from build123d import *

# Parameters (mm, degrees)
PRISM_DEPTH       = 2.4
PRISM001_DEPTH    = 2.4
CYLINDER012_R     = 1.25
CYLINDER012_DEPTH = 50
CYLINDER011_R     = 1.25
CYLINDER011_DEPTH = 50
CYLINDER007_R     = 6.75
CYLINDER007_DEPTH = 50
CYLINDER008_R     = 6.75
CYLINDER008_DEPTH = 50
BOX002_W          = 18
BOX002_H          = 18
BOX002_DEPTH      = 15
BOX003_W          = 18
BOX003_H          = 18
BOX003_DEPTH      = 15
CYLINDER004_R     = 11.2
CYLINDER004_DEPTH = 23
CYLINDER002_R     = 0.9
CYLINDER002_DEPTH = 19.75
ARRAY001_COUNT    = 10
CYLINDER006_R     = 10.5
CYLINDER006_DEPTH = 32
CYLINDER005_R     = 20
CYLINDER005_DEPTH = 15
FILLET003_R       = 1
CYLINDER029_R     = 1.25
CYLINDER029_DEPTH = 50
BOX009_W          = 16
BOX009_H          = 1
BOX009_DEPTH      = 15
CYLINDER030_R     = 1.25
CYLINDER030_DEPTH = 50
BOX010_W          = 16
BOX010_H          = 1
BOX010_DEPTH      = 15
FILLET010_R       = 0.9


with BuildPart() as prism:
    # Prism → Prism (new body)
    with BuildSketch(Plane(origin=(0, 28, 22.5), x_dir=(1, 0, 0), z_dir=(0, -1, 0))):
        Polygon((3.15, 0), (1.575, 2.72798), (-1.575, 2.72798), (-3.15, 0), (-1.575, -2.72798), (1.575, -2.72798), align=None)
    extrude(amount=PRISM_DEPTH)


with BuildPart() as prism001:
    # Prism001 → Prism001 (new body)
    with BuildSketch(Plane(origin=(0, -25.5, 22.5), x_dir=(1, 0, 0), z_dir=(0, -1, 0))):
        Polygon((3.15, 0), (1.575, 2.72798), (-1.575, 2.72798), (-3.15, 0), (-1.575, -2.72798), (1.575, -2.72798), align=None)
    extrude(amount=PRISM001_DEPTH)


with BuildPart() as cylinder011:
    # Cylinder012 → Cylinder012 (new body)
    with BuildSketch(Plane(origin=(0, 69, 22.5), x_dir=(1, 0, 0), z_dir=(0, -1, 0))):
        Circle(CYLINDER012_R)
    extrude(amount=CYLINDER012_DEPTH)


with BuildPart() as cylinder010:
    # Cylinder011 → Cylinder011 (new body)
    with BuildSketch(Plane(origin=(0, -16, 22.5), x_dir=(1, 0, 0), z_dir=(0, -1, 0))):
        Circle(CYLINDER011_R)
    extrude(amount=CYLINDER011_DEPTH)


with BuildPart() as cylinder007:
    # Cylinder007 → Cylinder007 (new body)
    with BuildSketch(Plane(origin=(-24, 19, 22.5), x_dir=(0, 0, -1), z_dir=(1, 0, 0))):
        Circle(CYLINDER007_R)
    extrude(amount=CYLINDER007_DEPTH)


with BuildPart() as cylinder008:
    # Cylinder008 → Cylinder008 (new body)
    with BuildSketch(Plane(origin=(-24, -19, 22.5), x_dir=(0, 0, -1), z_dir=(1, 0, 0))):
        Circle(CYLINDER008_R)
    extrude(amount=CYLINDER008_DEPTH)


with BuildPart() as cube002:
    # Box002 → Box002 (new body)
    with BuildSketch(Plane(origin=(-9, -29, 15), x_dir=(1, 0, 0), z_dir=(0, 0, 1))):
        with Locations((9, 9)):
            Rectangle(BOX002_W, BOX002_H)
    extrude(amount=BOX002_DEPTH)


with BuildPart() as cube003:
    # Box003 → Box003 (new body)
    with BuildSketch(Plane(origin=(-9, 11, 15), x_dir=(1, 0, 0), z_dir=(0, 0, 1))):
        with Locations((9, 9)):
            Rectangle(BOX003_W, BOX003_H)
    extrude(amount=BOX003_DEPTH)


with BuildPart() as cylinder004:
    # Cylinder004 → Cylinder004 (new body)
    with BuildSketch(Plane.XY):
        Circle(CYLINDER004_R)
    extrude(amount=CYLINDER004_DEPTH)


with BuildPart() as obj1:
    # Cylinder002 → Cylinder002 (new body)
    with BuildSketch(Plane(origin=(0, 0, 15), x_dir=(0, 0, -1), z_dir=(1, 0, 0))):
        Circle(CYLINDER002_R)
    extrude(amount=CYLINDER002_DEPTH)

    # Array001: obj1 ×10 about axis
    array001_axis = Axis((0, 0, 0), (0, 0, 1))


with BuildPart() as obj1_1:
    add(obj1.part)
    for i in range(1, ARRAY001_COUNT):
        add(obj1.part.rotate(array001_axis, i * 360 / ARRAY001_COUNT))

    # Cut002: cut Cylinder004
    add(cylinder004.part, mode=Mode.SUBTRACT)


with BuildPart() as cylinder006:
    # Cylinder006 → Cylinder006 (new body)
    with BuildSketch(Plane.XY):
        Circle(CYLINDER006_R)
    extrude(amount=CYLINDER006_DEPTH)


with BuildPart() as obj2:
    # Cylinder005 → Cylinder005 (new body)
    with BuildSketch(Plane.XY.offset(15)):
        Circle(CYLINDER005_R)
    extrude(amount=CYLINDER005_DEPTH)

    # Cut004: cut Cylinder006
    add(cylinder006.part, mode=Mode.SUBTRACT)

    # Fusion001: union obj1
    add(obj1_1.part)

    # Fusion002: union Cube002, Cube003
    add(cube002.part)
    add(cube003.part)

    # Cut005: cut Cylinder008
    add(cylinder008.part, mode=Mode.SUBTRACT)

    # Cut006: cut Cylinder007
    add(cylinder007.part, mode=Mode.SUBTRACT)

    # Fillet003
    fillet003_edges = [obj2.edges().sort_by_distance(p)[0] for p in [
        (-9, -17.860571, 29.576567),
        (-9, -17.860571, 15.423433),
        (-9, -29, 22.5),
        (-9, 17.860571, 15.423433),
        (-9, 17.860571, 29.576567),
        (9, -29, 22.5),
        (9, -17.860571, 29.576567),
        (9, -17.860571, 15.423433),
        (9, 17.860571, 29.576567),
        (9, 17.860571, 15.423433),
        (9, 29, 22.5),
        (-9, 29, 22.5),
    ]]
    fillet(fillet003_edges, radius=FILLET003_R)

    # Cut008: cut Cylinder010
    add(cylinder010.part, mode=Mode.SUBTRACT)

    # Cut009: cut Cylinder011
    add(cylinder011.part, mode=Mode.SUBTRACT)

    # Cut025: cut Prism001
    add(prism001.part, mode=Mode.SUBTRACT)

    # Cut026: cut Prism
    add(prism.part, mode=Mode.SUBTRACT)


with BuildPart() as cylinder020:
    # Cylinder029 → Cylinder029 (new body)
    with BuildSketch(Plane(origin=(0, 69, 22.5), x_dir=(1, 0, 0), z_dir=(0, -1, 0))):
        Circle(CYLINDER029_R)
    extrude(amount=CYLINDER029_DEPTH)


with BuildPart() as cut027:
    # Box009 → Box009 (new body)
    with BuildSketch(Plane(origin=(-8, 29, 15), x_dir=(1, 0, 0), z_dir=(0, 0, 1))):
        with Locations((8, 0.5)):
            Rectangle(BOX009_W, BOX009_H)
    extrude(amount=BOX009_DEPTH)

    # Cut027: cut Cylinder020
    add(cylinder020.part, mode=Mode.SUBTRACT)


with BuildPart() as cylinder021:
    # Cylinder030 → Cylinder030 (new body)
    with BuildSketch(Plane(origin=(0, 69, 22.5), x_dir=(1, 0, 0), z_dir=(0, -1, 0))):
        Circle(CYLINDER030_R)
    extrude(amount=CYLINDER030_DEPTH)


with BuildPart() as obj3:
    # Box010 → Box010 (new body)
    with BuildSketch(Plane(origin=(-8, 29, 15), x_dir=(1, 0, 0), z_dir=(0, 0, 1))):
        with Locations((8, 0.5)):
            Rectangle(BOX010_W, BOX010_H)
    extrude(amount=BOX010_DEPTH)

    # Cut028: cut Cylinder021
    add(cylinder021.part, mode=Mode.SUBTRACT)


with BuildPart() as obj3_1:
    # Cut028 placement: moved
    add(obj3.part.moved(Location((0, -59, 0))))

    # Fusion008: union obj2, Cut027
    add(obj2.part)
    add(cut027.part)

    # Fillet010
    fillet010_edges = [obj3_1.edges().sort_by_distance(p)[0] for p in [
        (-8, -30, 22.5),
        (8, -30, 22.5),
        (-8, 30, 22.5),
        (8, 30, 22.5),
    ]]
    fillet(fillet010_edges, radius=FILLET010_R)


solid = obj3_1.part
Check sheet for the modelled part. Datum: model origin and axes. Units: mm. A direction names the side the tool comes from. Round coordinates to 2 decimals unless told otherwise and drop trailing zeros. Loops run counter-clockwise (first coordinate to the right, second up) from the corner with the lowest first, then second, coordinate; pieces in that order, holes last. Notation, with made-up numbers: M -14.75,73.5 L 19.25,73.5 A26 ccw 19.25,97.5 Z; hole C 70.5,7 d7. An arc over 180 degrees is marked long. One line per item, written item: value.
(1) Thickness scan on line 1 (X direction, y = 29.05, z = 22.5); line 2 (Z direction, x = -2.5, y = -19); line 3 (Y direction, x = 0, z = 25). Record the ranges inside material, lowest first.
Computed values:
line 1: x = -8 to -1.25, 1.25 to 8
line 2: z = 15 to 15.75, 29.25 to 30
line 3: y = -30 to -27.9, -25.5 to -25.27, -12.73 to -10.5, 10.5 to 12.73, 25.27 to 25.6, 28 to 30
(2) Sectioned sample at C-C, the plane y = 26.5. Record the cut outline in (x, z) (3 decimals), then the cut area to 3 significant figures.
Computed values:
outline: M -9,15 L 9,15 L 9,30 L -9,30 Z; hole M -3.15,22.5 L -1.575,19.772 L 1.575,19.772 L 3.15,22.5 L 1.575,25.228 L -1.575,25.228 Z
area: 244 mm^2
(3) Depth check by flat-ended pin: pin 1 Ø1.9 at (x, y) = (0, 27.5) entering from -Z; pin 2 Ø4 at (x, z) = (13, 28.5) entering from -Y; pin 3 Ø1.5 at (x, z) = (0, 22.5) entering from -Y; pin 4 Ø8 at (y, z) = (-3, 20.5) entering from +X. Enter the tip coordinate at first touch or a pass-through.
Computed values:
pin 1: stops at z = 15
pin 2: stops at y = -16.68
pin 3: stops at y = -12.29
pin 4: stops at x = 20
(4) Sectioned sample at B-B, the plane y = 0. Record the cut outline in (x, z).
Computed values:
outline: M -20,15 L -19.75,15 L -19.75,14.1 L -11.2,14.1 L -11.2,15 L -10.5,15 L -10.5,30 L -20,30 Z; M 10.5,15 L 11.2,15 L 11.2,14.1 L 19.75,14.1 L 19.75,15 L 20,15 L 20,30 L 10.5,30 Z
(5) Release check for a two-part mould opening along Y. For faces 5 (the face through (9, 26, 22)), 6 (the face through (-2, 30, 22)), 7 (the face through (-4.8, -14.6, 14.1)) record: +Y half, -Y half, draft (parallel to the pull), parting line (faces both ways), or undercut.
Computed values:
face 5: draft
face 6: +Y half
face 7: undercut
(6) Sectioned sample at A-A, the plane x = 0. Record the cut outline in (y, z), then the cut area to 3 significant figures.
Computed values:
outline: M -30,15 L -10.5,15 L -10.5,30 L -30,30 L -30,23.75 L -27.9,23.75 L -27.9,25.23 L -25.5,25.23 L -25.5,24.32 A6.75 cw long -25.5,20.68 L -25.5,19.77 L -27.9,19.77 L -27.9,21.25 L -30,21.25 Z; M 10.5,15 L 30,15 L 30,21.25 L 28,21.25 L 28,19.77 L 25.6,19.77 L 25.6,21.08 A6.75 cw long 25.6,23.92 L 25.6,25.23 L 28,25.23 L 28,23.75 L 30,23.75 L 30,30 L 10.5,30 Z
area: 263 mm^2
(7) Sectioned sample at D-D, the plane y = -22. Record the cut outline in (x, z).
Computed values:
outline: M -9,15 L 9,15 L 9,16.45 L -9,16.45 Z; M -9,28.55 L 9,28.55 L 9,30 L -9,30 Z
(8) Access from +Z, -Z, +X, -X, +Y, -Y to the whole of each face (thin tool, end or side, straight path). Record for faces 1 (the face through (9, -26, 22)), 2 (the face through (-2.4, -26.7, 21.2)), 3 (the face through (-4.7, 14.6, 14.1)), 4 (the face through (-0.27, 29.01, 21.28)).
Computed values:
face 1: +Z, -Z, +X, -Y
face 2: none
face 3: -Z
face 4: +Y
